Could you check a few things on this model? Use its own coordinates, in mm. Face numbers are marked on the shaded views. A direction names the side the tool comes from. Coordinates: 2 decimals unless noted, no trailing zeros. Loops run counter-clockwise (first coordinate to the right, second up) from the corner with the lowest first, then second, coordinate; pieces in that order, holes last. Notation, with made-up numbers: (-30.5, -37.5) -> (-19.5, -37.5) arc R26 cw to (-19.5, -21.5) -> close; hole circle Ø6 at (54.25, 9.25). An arc over 180 degrees is marked (long way). One line per question, with ' | ' between items.
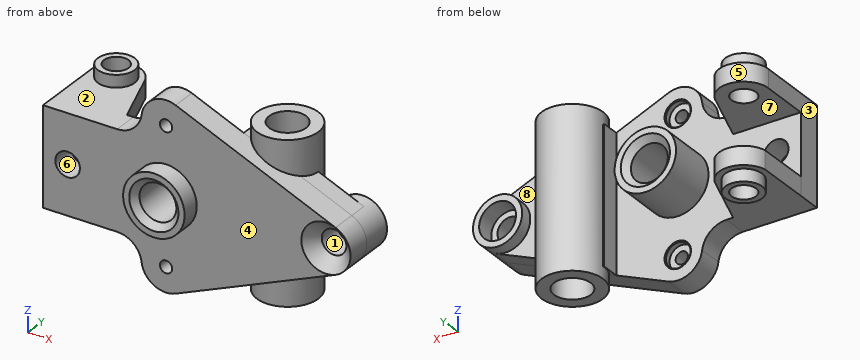
```python
from build123d import *

# Parameters (mm, degrees)
SKETCH4_R                               = 10
BOSS_EXTRUDE1_DEPTH                     = 20
SKETCH5_R                               = 10
BOSS_EXTRUDE2_DEPTH                     = 15
BOSS_EXTRUDE4_START                     = 10
SKETCH6_R                               = 15
SKETCH6_R_2                             = 10
BOSS_EXTRUDE4_DEPTH                     = 10
BOSS_EXTRUDE6_START                     = -15
SKETCH10_R                              = 10
BOSS_EXTRUDE6_DEPTH                     = 15
SKETCH11_R                              = 15
SKETCH11_R_2                            = 10
BOSS_EXTRUDE7_DEPTH                     = 10
CBORE_FOR_M10_HEX_HEAD_BOLT2_AT_2_COUNT = 2
CBORE_FOR_M10_HEX_HEAD_BOLT2_AT_2_PITCH = 462.374719531
CBORE_FOR_M10_HEX_HEAD_BOLT2_AT_3_COUNT = 2
CBORE_FOR_M10_HEX_HEAD_BOLT2_AT_3_PITCH = 110
BOSS_EXTRUDE8_DEPTH                     = 40
BOSS_EXTRUDE8_DEPTH_BACK                = 35
SKETCH12_R                              = 25
SKETCH19_R                              = 20
BOSS_EXTRUDE9_DEPTH                     = 25
BOSS_EXTRUDE10_DEPTH                    = 15
BOSS_EXTRUDE14_DEPTH                    = 65
BOSS_EXTRUDE14_DEPTH_BACK               = 65
SKETCH28_R                              = 25
SKETCH29_R                              = 15
CUT_EXTRUDE2_DEPTH                      = 181


with BuildPart() as part:
    # Sketch4 → Boss-Extrude1 (new body)
    with BuildSketch(Plane(origin=(0, 0, 0), x_dir=(1, 0, 0), z_dir=(0, 1, 0))):
        with BuildLine():
            Line((-77.28011811, -56.673598022), (-77.28011811, 23.326401978))
            Line((-77.28011811, 23.326401978), (-16.966387776, 23.326401978))
            ThreePointArc((-16.966387776, 23.326401978), (-3.737631221, 28.326401978), (2.876747057, 40.826401978))
            ThreePointArc((2.876747057, 40.826401978), (12.736944948, 55.656750215), (30.512681706, 56.745747))
            Line((30.512681706, 56.745747), (160.512681706, 1.745747))
            ThreePointArc((160.512681706, 1.745747), (172.71988189, -16.673598022), (160.512681706, -35.092943043))
            Line((160.512681706, -35.092943043), (30.512681706, -90.092943043))
            ThreePointArc((30.512681706, -90.092943043), (12.736944948, -89.003946259), (2.876747057, -74.173598022))
            ThreePointArc((2.876747057, -74.173598022), (-3.737631221, -61.673598022), (-16.966387776, -56.673598022))
            Line((-16.966387776, -56.673598022), (-77.28011811, -56.673598022))
        make_face()
        with Locations(Location((-57.28011811, -16.673598022, 0), (0, 0, 270))):
            Circle(SKETCH4_R, mode=Mode.SUBTRACT)
    extrude(amount=BOSS_EXTRUDE1_DEPTH)

    # Sketch5 → Boss-Extrude2 (add)
    with BuildSketch(Plane.XY.offset(56.673598022)):
        with BuildLine():
            Line((-77.28011811, 20), (-77.28011811, 60))
            ThreePointArc((-77.28011811, 60), (-60.595178298, 79.723345962), (-38.379080515, 66.538407896))
            Line((-38.379080515, 66.538407896), (-22.28011811, 20))
            Line((-22.28011811, 20), (-77.28011811, 20))
        make_face()
        with Locations((-57.28011811, 60)):
            Circle(SKETCH5_R, mode=Mode.SUBTRACT)
    extrude(amount=-BOSS_EXTRUDE2_DEPTH)

    # Sketch6 → Boss-Extrude4 (add)
    with BuildSketch(Plane.XY.offset(56.673598022).offset(BOSS_EXTRUDE4_START)):
        with Locations(Location((-57.28011811, 60, 0), (0, 0, 180))):
            Circle(SKETCH6_R)
        with Locations((-57.28011811, 60)):
            Circle(SKETCH6_R_2, mode=Mode.SUBTRACT)
    extrude(amount=-BOSS_EXTRUDE4_DEPTH)

    # Sketch10 → Boss-Extrude6 (add)
    with BuildSketch(Plane(origin=(0, 0, -23.326401978), x_dir=(-1, 0, 0), z_dir=(0, 0, -1)).offset(BOSS_EXTRUDE6_START)):
        with BuildLine():
            Line((22.28011811, 20), (38.379080515, 66.538407896))
            ThreePointArc((38.379080515, 66.538407896), (58.842761472, 79.938860191), (76.96898439, 63.514049605))
            Line((76.96898439, 63.514049605), (77.28011811, 20))
            Line((77.28011811, 20), (22.28011811, 20))
        make_face()
        with Locations(Location((57.28011811, 60, 0), (0, 0, 180))):
            Circle(SKETCH10_R, mode=Mode.SUBTRACT)
    extrude(amount=BOSS_EXTRUDE6_DEPTH)

    # Sketch11 → Boss-Extrude7 (add)
    with BuildSketch(Plane(origin=(0, 0, -23.326401978), x_dir=(-1, 0, 0), z_dir=(0, 0, -1))):
        with Locations((57.28011811, 60)):
            Circle(SKETCH11_R)
        with Locations(Location((57.28011811, 60, 0), (0, 0, 180))):
            Circle(SKETCH11_R_2, mode=Mode.SUBTRACT)
    extrude(amount=BOSS_EXTRUDE7_DEPTH)

    # Sketch16 → CBORE for M10 Hex Head Bolt2 (revolve, cut)
    with BuildSketch(Plane(origin=(22.71988189, 20, 71.673598022), x_dir=(0, 0, 1), z_dir=(1, 0, 0))):
        Polygon((0, 0), (0, 20), (5, 20), (5, 5), (10, 5), (10, 0.639813469), (10.7625, 0), align=None)
    cbore_for_m10_hex_head_bolt2 = revolve(axis=Axis((22.71988189, 26.35, 71.673598022), (0, -1, 0)), mode=Mode.SUBTRACT)

    # CBORE for M10 Hex Head Bolt2 at 2: CBORE for M10 Hex Head Bolt2 ×2
    with Locations(*[Vector(-0.05491608922209683, 0, -0.9984909729910185) * (i * CBORE_FOR_M10_HEX_HEAD_BOLT2_AT_2_PITCH) for i in range(1, CBORE_FOR_M10_HEX_HEAD_BOLT2_AT_2_COUNT)]):
        add(cbore_for_m10_hex_head_bolt2, mode=Mode.SUBTRACT)

    # CBORE for M10 Hex Head Bolt2 at 3: CBORE for M10 Hex Head Bolt2 ×2
    with Locations(*[(0, 0, -i * CBORE_FOR_M10_HEX_HEAD_BOLT2_AT_3_PITCH) for i in range(1, CBORE_FOR_M10_HEX_HEAD_BOLT2_AT_3_COUNT)]):
        add(cbore_for_m10_hex_head_bolt2, mode=Mode.SUBTRACT)

    # Sketch12 → Boss-Extrude8 (add, two sides: drawn at the far end of the back side and taken through both)
    with BuildSketch(Plane(origin=(0, 20, 0), x_dir=(1, 0, 0), z_dir=(0, 1, 0)).offset(-BOSS_EXTRUDE8_DEPTH_BACK)):
        with Locations(Location((22.71988189, -16.673598022, 0), (0, 0, 270))):
            Circle(SKETCH12_R)
    extrude(amount=BOSS_EXTRUDE8_DEPTH + BOSS_EXTRUDE8_DEPTH_BACK)

    # Sketch18 → CSK for M10 Countersunk Flat Head Screw1 (revolve, cut)
    with BuildSketch(Plane(origin=(22.71988189, 60, 16.673598022), x_dir=(0, 0, 1), z_dir=(1, 0, 0))):
        Polygon((0, 0), (0, 75), (20, 75), (15, 70), (15, 5), (20, 0), align=None)
    revolve(axis=Axis((22.71988189, 66.35, 16.673598022), (0, -1, 0)), mode=Mode.SUBTRACT)

    # Sketch19 → Boss-Extrude9 (add)
    with BuildSketch(Plane(origin=(0, 20, 0), x_dir=(1, 0, 0), z_dir=(0, 1, 0))):
        with Locations(Location((152.71988189, -16.673598022, 0), (0, 0, 67.067899562))):
            Circle(SKETCH19_R)
    extrude(amount=BOSS_EXTRUDE9_DEPTH)

    # Sketch20 → CBORE for M10 Hex Head Bolt3 (revolve, cut)
    with BuildSketch(Plane(origin=(152.71988189, 45, 16.673598022), x_dir=(0, 0, 1), z_dir=(1, 0, 0))):
        Polygon((0, 0), (0, 45), (20, 45), (10, 35), (10, 15), (15, 15), (15, 0), align=None)
    revolve(axis=Axis((152.71988189, 51.35, 16.673598022), (0, -1, 0)), mode=Mode.SUBTRACT)

    # Sketch23 → Boss-Extrude10 (add)
    with BuildSketch(Plane(origin=(0, 20, 0), x_dir=(1, 0, 0), z_dir=(0, 1, 0))):
        with BuildLine():
            ThreePointArc((160.512681706, -35.092943043), (132.71988189, -16.673598022), (160.512681706, 1.745747))
            Line((160.512681706, 1.745747), (72.71988189, 38.888854614))
            Line((72.71988189, 38.888854614), (72.71988189, -72.236050658))
            Line((72.71988189, -72.236050658), (160.512681706, -35.092943043))
        make_face()
    extrude(amount=BOSS_EXTRUDE10_DEPTH)

    # Sketch28 → Boss-Extrude14 (add, two sides: drawn at the far end of the back side and taken through both)
    with BuildSketch(Plane(origin=(0, 0, 16.673598022), x_dir=(-1, 0, 0), z_dir=(0, 0, -1)).offset(-BOSS_EXTRUDE14_DEPTH_BACK)):
        with Locations((-98.511863988, 35)):
            Circle(SKETCH28_R)
    extrude(amount=BOSS_EXTRUDE14_DEPTH + BOSS_EXTRUDE14_DEPTH_BACK)

    # Sketch29 → Cut-Extrude2 (cut)
    with BuildSketch(Plane(origin=(0, 0, -48.326401978), x_dir=(-1, 0, 0), z_dir=(0, 0, -1))):
        with Locations((-98.511863988, 35)):
            Circle(SKETCH29_R)
    extrude(amount=-CUT_EXTRUDE2_DEPTH, mode=Mode.SUBTRACT)


solid = part.part
```
Q1. Imagine slicing it at B-B on x = 67. Write out the boundary of the cut face in (y, z), plus the area to 3 significant figures.
Values follow:
outline: (0, -41.31) -> (20, -41.31) -> (20, 74.66) -> (0, 74.66) -> close | area: 2,320 mm2
Q2. For the marked faces 4, 5, 6, 7 and 8, which set-ups out of +Z, -Z, +X, -X, +Y, -Y let a thin tool reach every point of the face, with its end or its side?
Values follow:
face 4: -Y | face 5: +Z, -Z, +Y | face 6: +Y, -Y | face 7: -X, +Y | face 8: +Y
Q3. For pin 1 (4 mm diameter, centred on y = 34, z = -1, fed in from -X); pin 2 (24 mm diameter, centred on x = 158, z = 18, fed in from +Y); pin 3 (13 mm diameter, centred on x = 22.72, z = -38.33, fed in from -Y); pin 4 (16.5 mm diameter, centred on y = 28, z = 10, fed in from -X), each with a flat end and sliding along its axis, tell me the tip position at first contact or that it passes through.
Values follow:
pin 1: stops at x = 3.24 | pin 2: stops at y = 45 | pin 3: stops at y = 0 | pin 4: stops at x = -77.28
Q4. We'd pull the mould along Z, two halves only. Please class the marked faces 1, 2 and 3: released by +Z, released by -Z, zero draft, split by the parting line, or undercut.
Values follow:
face 1: undercut | face 2: released by +Z | face 3: zero draft
Q5. Please list where these lines run through material, in increasing order: L1, parallel to X at y = 22, z = 54; L2, parallel to X at y = 29, z = 46.5; L3, parallel to Y at x = 131.5, z = -8.5. Write a range as [from, to].
Values follow:
L1: x = [-77.28, -22.97], [72.72, 91.03], [106, 119.87] | L2: x = [-77.28, -25.39], [72.72, 84.76], [112.26, 133.55] | L3: y = [0, 35]
Q6. Imagine slicing it at A-A on z = 15.5. Give the number of separate pieces and of enclosed holes in the cut face, plus the area to 3 significant figures.
Values follow:
separate pieces: 4 | enclosed holes: 1 | area: 6,080 mm2
